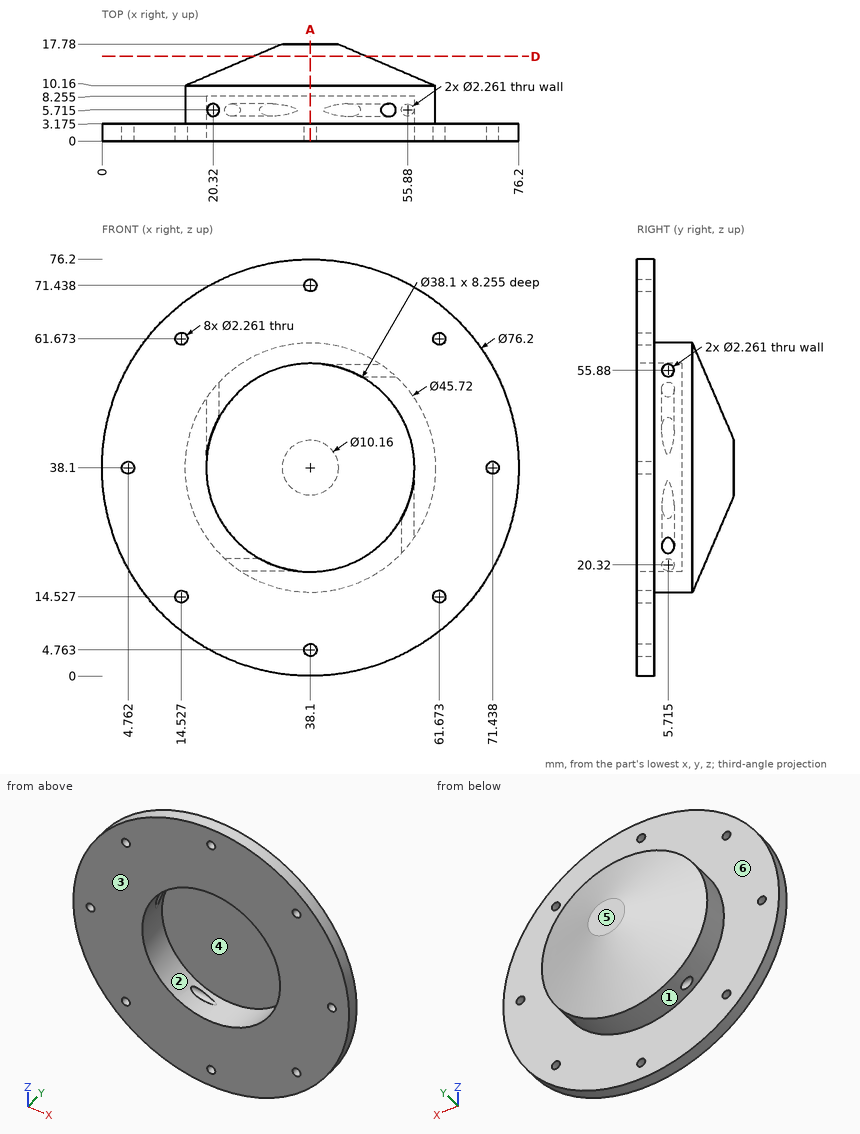
Drawing for the job (mm, zero at the part's lowest x, y, z). A direction names the side the tool comes from. Coordinates: 2 decimals unless noted, no trailing zeros. Loops run counter-clockwise (first coordinate to the right, second up) from the corner with the lowest first, then second, coordinate; pieces in that order, holes last. Notation, with made-up numbers: (20.5, -7.75) - (60.5, -7.75) arc R4 ccw to (60.5, -3.75) - close; hole circle Ø2 at (46, 52.5). An arc over 180 degrees is marked (long way). Return JSON: item names as keys, results as strings.
1. Mould opens along X. For the marked faces 1, 2 and 3 say: released by +X, released by -X, zero draft, split by the parting line, or undercut.
Result:
{"face 1": "split by the parting line", "face 2": "undercut", "face 3": "zero draft"}
2. Band-saw the part on D-D (y = 15.5). Give the cut face in (x, z).
Result:
{"outline": "circle Ø20.8 at (38.1, 38.1)"}
3. Probe L1, parallel to Z at x = 38.1, y = 1.05; L2, parallel to Y at x = 67.5, z = 59 (1 decimal); L3, parallel to X at y = 10, z = 39. List the from-to ranges inside material, lowest first. Write a range as from..to.
Result:
{"L1": "z = 0..3.63, 5.89..19.05, 57.15..70.31, 72.57..76.2", "L2": "y = 0..3.2", "L3": "x = 15.26..60.94"}
4. 3-axis set-ups, long thin cutter, end or side, ignore diameter. For the marked faces 4, 5 and 6: which of +Z, -Z, +X, -X, +Y, -Y reach the whole face in a straight line?
Result:
{"face 4": "-Y", "face 5": "+Z, -Z, +X, -X, +Y", "face 6": "+Y"}
5. Drop flat-ended pins along their axis: pin 1 (5 mm diameter, centred on x = 25.5, z = 43.5, fed in from +Y); pin 2 (2 mm diameter, centred on x = 61.67, z = 14.53, fed in from -Y); pin 3 (3 mm diameter, centred on x = 20.32, y = 5.715, fed in from -Z); pin 4 (2.5 mm diameter, centred on y = 5.715, z = 20.32, fed in from +X). Give the stop position or say it passes through.
Result:
{"pin 1": "stops at y = 15.15", "pin 2": "passes through", "pin 3": "stops at z = 22.05", "pin 4": "stops at x = 53.89"}
6. Band-saw the part on A-A (x = 38.1). State how many separate pieces and enclosed holes the cut face has.
Result:
{"separate pieces": "3", "enclosed holes": "0"}
